Verification items for the finished model (mm, model axes). Give positions to 0.01 mm unless a question says otherwise; leave off trailing zeros. Loops run counter-clockwise (first coordinate to the right, second up) from the corner with the lowest first, then second, coordinate; pieces in that order, holes last. Notation, with made-up numbers: (13.5, 63.5) - (54.5, 63.5) arc R14 ccw to (54.5, 88.5) - close; hole circle Ø3 at (-34.75, 68.25). An arc over 180 degrees is marked (long way). One line per item, written item: value. Start each with the question number.
1. Gauge pin test, flat ends, axial feed: pin 1 (4 mm diameter, centred on x = -11.2, y = 15, fed in from +Z); pin 2 (4 mm diameter, centred on x = -11, y = -14.5, fed in from +Z); pin 3 (3 mm diameter, centred on x = -11.2, y = -15, fed in from +Z) (3 decimals). Record the tip position at first contact, or that the pin passes through.
2. Scan lines: L1, parallel to Y at x = -12.25, z = 0.9; L2, parallel to Y at x = 11, z = 1.9; L3, parallel to X at y = 13, z = 2.85. Record each from-to range of solid material in increasing order. Write a range as [from, to].
3. Sectioned sample at B-B (z = 0.55). Record the cut outline in (x, y), plus the area to 3 significant figures.
4. Sectioned sample at A-A (x = -11.2). Record the cut outline in (y, z).
5. Mould release check, pull along Y, two halves, no side actions. Record for faces 1 (the cylindrical face through (12.63, 18.36, 1.52)), 2 (the cylindrical face through (12.56, -18.43, 1.52)), 3 (the cylindrical face through (-11.428, -13.265, 1.014)): pulls with the +Y half, pulls with the -Y half, needs draft (parallel to the pull), parting line crosses it, or undercut.
from build123d import *

# Parameters (mm, degrees)
SZKIC1_W                    = 28.4
SZKIC1_H                    = 40
DODANIE_WYCI_GNI_CIE1_DEPTH = 3
ZAOKR_GLENIE1_R             = 5
SZKIC2_R                    = 1.75
WYTNIJ_WYCI_GNI_CIE1_DEPTH  = 3
SFAZOWANIE1_SIZE            = 1
WYTNIJ_WYCI_GNI_CIE2_DEPTH  = 3


with BuildPart() as part:
    # Szkic1 → Dodanie-wyciągnięcie1 (new body)
    with BuildSketch(Plane.XY):
        Rectangle(SZKIC1_W, SZKIC1_H)
    extrude(amount=DODANIE_WYCI_GNI_CIE1_DEPTH)

    # Zaokrąglenie1
    zaokr_glenie1_edges = [part.edges().sort_by_distance(p)[0] for p in [
        (14.2, -20, 1.5),
        (-14.2, -20, 1.5),
        (-14.2, 20, 1.5),
        (14.2, 20, 1.5),
    ]]
    fillet(zaokr_glenie1_edges, radius=ZAOKR_GLENIE1_R)

    # Szkic2 → Wytnij-wyciągnięcie1 (cut)
    with BuildSketch(Plane.XY.offset(3)):
        with Locations((-11.2, 15)):
            Circle(SZKIC2_R)
        with Locations((11.2, 15)):
            Circle(SZKIC2_R)
        with Locations((-11.2, -15)):
            Circle(SZKIC2_R)
        with Locations((11.2, -15)):
            Circle(SZKIC2_R)
    extrude(amount=-WYTNIJ_WYCI_GNI_CIE1_DEPTH, mode=Mode.SUBTRACT)

    # Sfazowanie1
    sfazowanie1_edges = [part.edges().sort_by_distance(p)[0] for p in [
        (9.45, 15, 3),
        (-12.95, -15, 3),
        (9.45, -15, 3),
        (-12.95, 15, 3),
    ]]
    chamfer(sfazowanie1_edges, length=SFAZOWANIE1_SIZE)

    # Szkic3 → Wytnij-wyciągnięcie2 (cut)
    with BuildSketch(Plane.XY.offset(3)):
        with BuildLine():
            Line((-14.2, 15), (-14.2, -15))
            ThreePointArc((-14.2, -15), (-12.735533906, -18.535533906), (-9.2, -20))
            Line((-9.2, -20), (9.2, -20))
            ThreePointArc((9.2, -20), (12.735533906, -18.535533906), (14.2, -15))
            Line((14.2, -15), (14.2, 15))
            ThreePointArc((14.2, 15), (12.735533906, 18.535533906), (9.2, 20))
            Line((9.2, 20), (-9.2, 20))
            ThreePointArc((-9.2, 20), (-12.735533906, 18.535533906), (-14.2, 15))
        make_face()
        with BuildLine():
            Line((9.2, 19.8), (-9.2, 19.8))
            ThreePointArc((-9.2, 19.8), (-12.59411255, 18.39411255), (-14, 15))
            Line((-14, 15), (-14, -15))
            ThreePointArc((-14, -15), (-12.59411255, -18.39411255), (-9.2, -19.8))
            Line((-9.2, -19.8), (9.2, -19.8))
            ThreePointArc((9.2, -19.8), (12.59411255, -18.39411255), (14, -15))
            Line((14, -15), (14, 15))
            ThreePointArc((14, 15), (12.59411255, 18.39411255), (9.2, 19.8))
        make_face(mode=Mode.SUBTRACT)
    extrude(amount=-WYTNIJ_WYCI_GNI_CIE2_DEPTH, mode=Mode.SUBTRACT)


solid = part.part
Results are:
1. pin 1: stops at z = 2.25
1. pin 2: stops at z = 2.79
1. pin 3: passes through
2. L1: y = [-18.71, -16.4], [-13.6, 13.6], [16.4, 18.71]
2. L2: y = [-19.45, -16.74], [-13.26, 13.26], [16.74, 19.45]
2. L3: x = [-14, -12.86], [-9.54, 9.54], [12.86, 14]
3. outline: (-14, -15) arc R4.8 ccw to (-9.2, -19.8) - (9.2, -19.8) arc R4.8 ccw to (14, -15) - (14, 15) arc R4.8 ccw to (9.2, 19.8) - (-9.2, 19.8) arc R4.8 ccw to (-14, 15) - close; hole circle Ø3.5 at (-11.2, -15); hole circle Ø3.5 at (-11.2, 15); hole circle Ø3.5 at (11.2, -15); hole circle Ø3.5 at (11.2, 15)
3. area: 1,050 mm^2
4. outline: (-19.36, 0) - (-16.75, 0) - (-16.75, 2) - (-17.75, 3) - (-19.36, 3) - close; (-13.25, 0) - (13.25, 0) - (13.25, 2) - (12.25, 3) - (-12.25, 3) - (-13.25, 2) - close; (16.75, 0) - (19.36, 0) - (19.36, 3) - (17.75, 3) - (16.75, 2) - close
5. face 1: pulls with the +Y half
5. face 2: pulls with the -Y half
5. face 3: undercut
